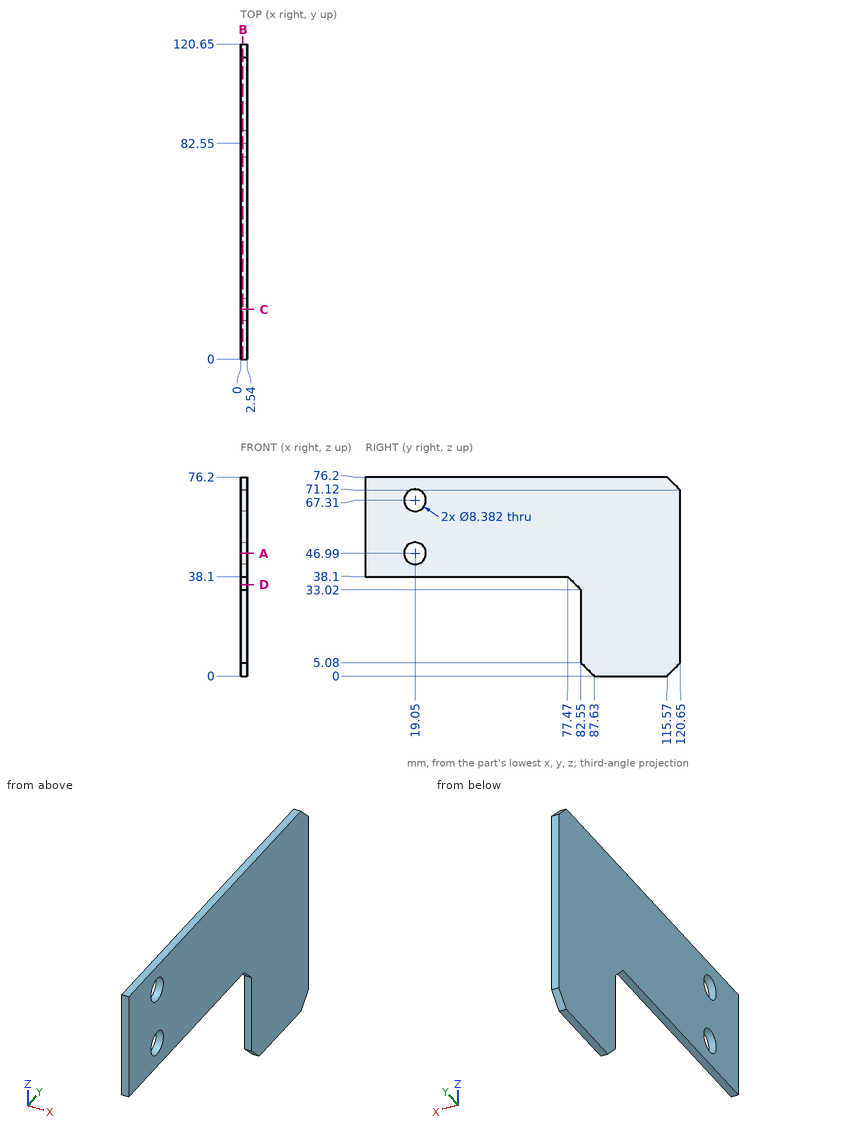
Part print with two shaded views. Sizes in mm from the minimum x, y, z corner. Round coordinates to 2 decimals unless told otherwise and drop trailing zeros. Write each loop counter-clockwise with the first axis right and the second up, starting at its lowest first coordinate (ties: lowest second). Pieces come first, ordered by that corner, then holes. Notation, with made-up numbers: (-1, -4.75) -> (16, -4.75) arc R31 ccw to (16, 20.25) -> close; hole circle Ø8 at (-17, 16). An arc over 180 degrees is marked (long way). Put each result on its own line as item: value.
Item 1: Slice it at B-B, the plane x = 0.8. Give the cut face in (y, z).
Here are the results:
outline: (0, 38.1) -> (77.47, 38.1) -> (82.55, 33.02) -> (82.55, 5.08) -> (87.63, 0) -> (115.57, 0) -> (120.65, 5.08) -> (120.65, 71.12) -> (115.57, 76.2) -> (0, 76.2) -> close; hole circle Ø8.38 at (19.05, 46.99); hole circle Ø8.38 at (19.05, 67.31)
Item 2: Slice it at D-D, the plane z = 35. Give the cut face in (x, y).
Here are the results:
outline: (0, 80.57) -> (2.54, 80.57) -> (2.54, 120.65) -> (0, 120.65) -> close
Item 3: Flat gauge pins, fed straight in: P1, Ø0.8, axis at x = 1.5, y = 35, coming from the -Z side; P2, Ø1.5, axis at x = 2, z = 33.5, coming from the -Y side. Where does each tip first touch, or does it go through?
Here are the results:
P1: stops at z = 38.1
P2: stops at y = 81.32
Item 4: Slice it at A-A, the plane z = 46.99. Give the cut face in (x, y).
Here are the results:
outline: (0, 0) -> (2.54, 0) -> (2.54, 14.86) -> (0, 14.86) -> close; (0, 23.24) -> (2.54, 23.24) -> (2.54, 120.65) -> (0, 120.65) -> close
Item 5: Wall check: probe 1 along Y at (x, z) = (0.65, 46.99); probe 2 along Y at (x, z) = (2.2, 27.5); probe 3 along Z at (x, y) = (0.3, 22.5). Give the ranges that are in metal, low to high. Write a range as from..to.
Here are the results:
probe 1: y = 0..14.86, 23.24..120.65
probe 2: y = 82.55..120.65
probe 3: z = 38.1..44.61, 49.37..64.93, 69.69..76.2
Item 6: Slice it at C-C, the plane y = 19.05. Give the cut face in (x, z), plus the area to 3 significant figures.
Here are the results:
outline: (0, 38.1) -> (2.54, 38.1) -> (2.54, 42.8) -> (0, 42.8) -> close; (0, 51.18) -> (2.54, 51.18) -> (2.54, 63.12) -> (0, 63.12) -> close; (0, 71.5) -> (2.54, 71.5) -> (2.54, 76.2) -> (0, 76.2) -> close
area: 54.2 mm^2
